Study the drawing (mm; zero at the part's minimum x, y, z) and answer. Coordinates: 2 decimals unless noted, no trailing zeros. Order: outer loops, then holes, each group sorted by start corner. A loop starts at its lowest first (then second) coordinate and runs counter-clockwise, first axis right, second up. Notation, with made-up numbers: (68.25, 51) - (109.25, 51) arc R19 cw to (109.25, 77) - close; hole circle Ø11 at (35, 52). An arc over 180 degrees is marked (long way). Write item = value, one per line.
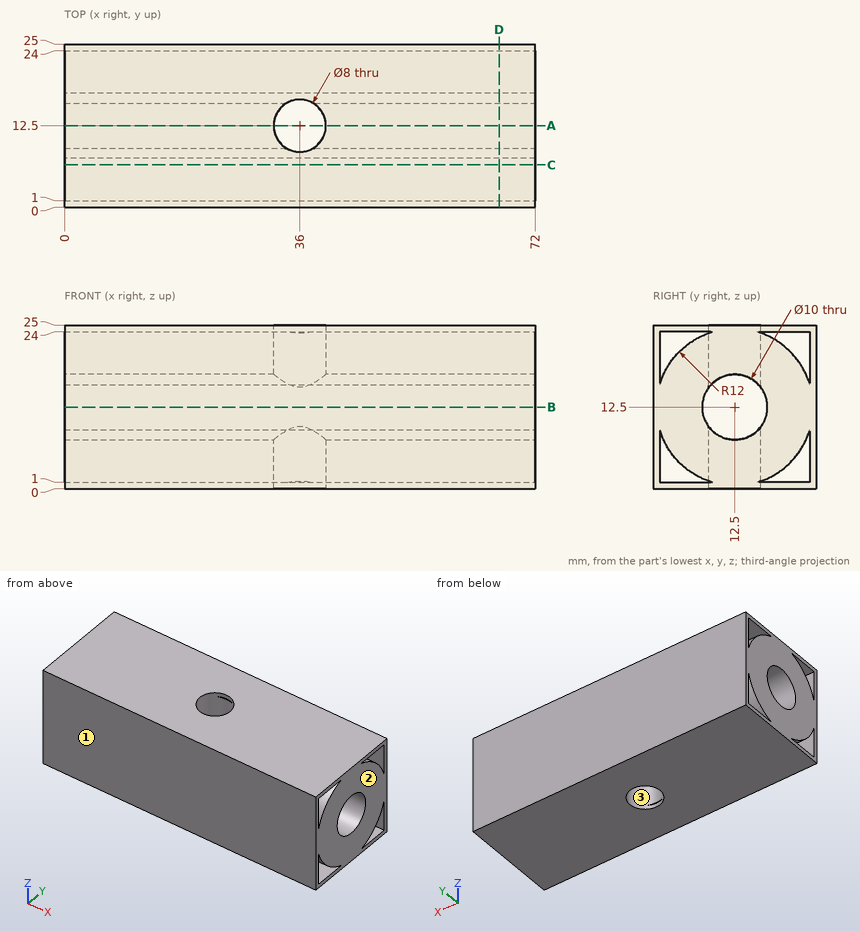
1) The part is cut by section C-C (y = 6.5). Determine the outline of the cut face in (x, z).
Returned:
outline = (0, 0) - (72, 0) - (72, 1) - (0, 1) - close; (0, 2.11) - (72, 2.11) - (72, 22.89) - (0, 22.89) - close; (0, 24) - (72, 24) - (72, 25) - (0, 25) - close
2) Straight lines are drawn through the part: line 1 along Y through (x, z) = (21, 12.5); line 2 along Y through (x, z) = (36, 21.5); line 3 along X through (y, z) = (12.5, 2). For each, find the intervals that lie inside material, in ascending order. Write a range as from..to.
Returned:
line_1 = 0..7.5, 17.5..25
line_2 = 0..1, 4.56..8.5, 16.5..20.44, 24..25
line_3 = 0..32, 40..72
3) The part is cut by section A-A (y = 12.5). Determine the outline of the cut face in (x, z), and give its area (3 significant figures).
Returned:
outline = (0, 0) - (32, 0) - (32, 7.5) - (0, 7.5) - close; (0, 17.5) - (32, 17.5) - (32, 25) - (0, 25) - close; (40, 0) - (72, 0) - (72, 7.5) - (40, 7.5) - close; (40, 17.5) - (72, 17.5) - (72, 25) - (40, 25) - close
area = 960 mm^2
4) Determine the mould class of the marked faces 1, 2 and 3 for opening direction X: pulls with the +X half, pulls with the -X half, needs draft (parallel to the pull), parting line crosses it, or undercut.
Returned:
face_1 = needs draft
face_2 = pulls with the +X half
face_3 = undercut
5) The part is cut by section D-D (x = 66.5). Determine the outline of the cut face in (y, z), and give its area (3 significant figures).
Returned:
outline = (0, 0) - (25, 0) - (25, 25) - (0, 25) - close; hole (1, 1) - (9.07, 1) arc R12 cw to (1, 9.07) - close; hole (1, 15.93) arc R12 cw to (9.07, 24) - (1, 24) - close; hole circle Ø10 at (12.5, 12.5); hole (15.93, 1) - (24, 1) - (24, 9.07) arc R12 cw to start; hole (15.93, 24) arc R12 cw to (24, 15.93) - (24, 24) - close
area = 461 mm^2
6) The part is cut by section B-B (z = 12.5). Determine the outline of the cut face in (x, y), and give its area (3 significant figures).
Returned:
outline = (0, 0) - (72, 0) - (72, 7.5) - (0, 7.5) - close; (0, 17.5) - (72, 17.5) - (72, 25) - (0, 25) - close
area = 1,080 mm^2
7) Flat-ended cylindrical pins translate along their axes: pin 1 Ø3 at (x, z) = (20.5, 20) entering from -Y; pin 2 Ø9 at (y, z) = (12.5, 12.5) entering from +X. Find the tip coordinate at first contact, or state that the pin passes through.
Returned:
pin_1 = 0
pin_2 = through
